Check sheet for the drawn part. Datum: minimum x, y, z corner. Units: mm. Give positions to 0.01 mm unless a question says otherwise; leave off trailing zeros. Write each loop counter-clockwise with the first axis right and the second up, starting at its lowest first coordinate (ties: lowest second). Pieces come first, ordered by that corner, then holes. Notation, with made-up numbers: (20, 15) - (55, 15) arc R32 cw to (55, 42) - close; hole circle Ø7 at (-27, 86.5). An arc over 180 degrees is marked (long way). One line per question, with ' | ' between items. Start each with the question number.
Q1. Section check C-C on x = 10.75. Record the boundary of the cut face in (y, z).
Q2. Section check B-B on y = 0.5. Record the boundary of the cut face in (x, z).
Q3. Section check A-A on x = 7. Record the boundary of the cut face in (y, z), and give its area (4 significant figures).
Q4. Thickness scan on L1, parallel to X at y = 1.3, z = 12.5; L2, parallel to Z at x = 11.25, y = 1.35; L3, parallel to Z at x = 3.75, y = 0.6. Record the ranges inside material, lowest first. Write a range as [from, to].
Q5. Gauge pin test, flat ends, axial feed: P1, Ø1, axis at x = 8.5, z = 8, coming from the -Y side; P2, Ø0.8, axis at y = 0.5, z = 47, coming from the +X side; P3, Ø0.8, axis at y = 0.5, z = 62.5, coming from the +X side. Record the tip position at first contact, or that the pin passes through.
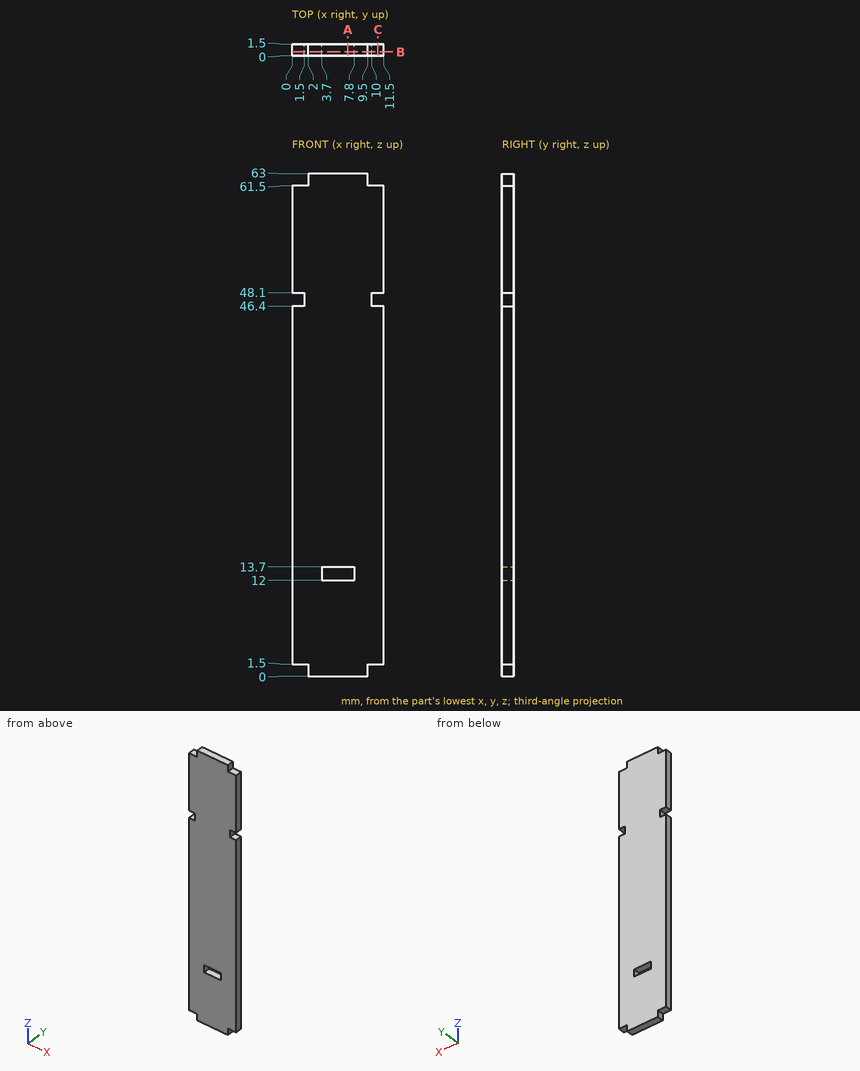
Working result:
1) outline: (0, 1.5) - (1.5, 1.5) - (1.5, 46.4) - (0, 46.4) - close; (0, 48.1) - (1.5, 48.1) - (1.5, 61.5) - (0, 61.5) - close
2) outline: (0, 1.5) - (2, 1.5) - (2, 0) - (9.5, 0) - (9.5, 1.5) - (11.5, 1.5) - (11.5, 46.4) - (10, 46.4) - (10, 48.1) - (11.5, 48.1) - (11.5, 61.5) - (9.5, 61.5) - (9.5, 63) - (2, 63) - (2, 61.5) - (0, 61.5) - (0, 48.1) - (1.5, 48.1) - (1.5, 46.4) - (0, 46.4) - close; hole (3.7, 12) - (7.8, 12) - (7.8, 13.7) - (3.7, 13.7) - close
3) outline: (0, 0) - (1.5, 0) - (1.5, 12) - (0, 12) - close; (0, 13.7) - (1.5, 13.7) - (1.5, 63) - (0, 63) - close | area: 91.95 mm2
4) L1: x = [0, 3.7], [7.8, 11.5] | L2: z = [1.5, 46.4], [48.1, 61.5] | L3: z = [0, 12], [13.7, 63]
5) P1: stops at y = 0 | P2: stops at x = 10 | P3: stops at x = 9.5
